from build123d import *

# Parameters (mm, degrees)
SKETCH001_R     = 6
POCKET_DEPTH    = 5.020854
CHAMFER_SIZE    = 0.25
CHAMFER001_SIZE = 1


with BuildPart() as pocket:
    # Sketch003 → Revolution001 (revolve)
    with BuildSketch(Plane.XZ):
        Polygon((0, -4.019854), (5, -2.2), (5, 1), (0, 1), align=None)
    revolve(axis=Axis((0, 0, 0), (0, 0, 1)))

    # Sketch001 → Pocket (cut, through all)
    with BuildSketch(Plane(origin=(0, 0, 1), x_dir=(-1, 0, 0), z_dir=(0, 0, 1))):
        Circle(SKETCH001_R)
        Polygon((-1.443376, 2.5), (1.443376, 2.5), (2.886751, 0), (1.443376, -2.5), (-1.443376, -2.5), (-2.886751, 0), align=None, mode=Mode.SUBTRACT)
    extrude(amount=-POCKET_DEPTH, mode=Mode.SUBTRACT)


with BuildPart() as chamfer001:
    # Sketch → Revolution (revolve)
    with BuildSketch(Plane.XZ):
        Polygon((2.88675, 0), (6.719999, 0), (3, -3.72), (3, -12), (0, -12), (0, -2.886753), align=None)
    revolve(axis=Axis((0, 0, 0), (0, 0, 1)))

    # Cut: cut Pocket
    add(pocket.part, mode=Mode.SUBTRACT)

    # Chamfer
    chamfer_edges = [chamfer001.edges().sort_by_distance(p)[0] for p in [
        (-6.719999, 0, 0),
    ]]
    chamfer(chamfer_edges, length=CHAMFER_SIZE)

    # Chamfer001
    chamfer001_edges = [chamfer001.edges().sort_by_distance(p)[0] for p in [
        (-3, 0, -12),
    ]]
    chamfer(chamfer001_edges, length=CHAMFER001_SIZE)


solid = chamfer001.part
Could you check a few things on this model? Use its own coordinates, in mm. A direction names the side the tool comes from. Give positions to 0.01 mm unless a question says otherwise; leave off trailing zeros. Order: outer loops, then holes, each group sorted by start corner. A loop starts at its lowest first (then second) coordinate and runs counter-clockwise, first axis right, second up. Notation, with made-up numbers: (71, 51.25) - (118, 51.25) arc R25 ccw to (118, 72.25) - close; hole circle Ø2 at (61.5, 43). An arc over 180 degrees is marked (long way). One line per question, with ' | ' between items. Start each with the question number.
Item 1: I'm going to push flat-ended pins straight in: pin 1 Ø4 at (y, z) = (-0.5, -10) entering from -X; pin 2 Ø1 at (y, z) = (2, -1.5) entering from -X; pin 3 Ø1.5 at (x, z) = (2, -3.5) entering from -Y. Where does each tip first touch, or does it pass through?
Item 2: I want a section at B-B on z = -9.75. Write out the boundary of the cut face in (x, y).
Item 3: I want a section at A-A on z = -2.25. Write out the boundary of the cut face in (x, y).
Item 4: For faces 1 (the flat face through (-2.175, 1.233, -1.533)), 2 (the cylindrical face through (-3, 0, -7)), 3 (the flat face through (-3, -1, 0)), which set-ups out of +Z, -Z, +X, -X, +Y, -Y let a thin tool reach every point of the face, with its end or its side?
Item 5: I need wall thicknesses on probe 1 along X at (y, z) = (-0.25, -1.75); probe 2 along Y at (x, z) = (0, -10.5); probe 3 along Z at (x, y) = (-3.75, 0). Which ranges of each line are inside material? Lowest first, please. Write a range as [from, to].
Item 6: Thinking about a two-plate mould opening in X: for faces 4 (the flat face through (0, 0, -12)), 5 (the conical face through (0.172, 0.054, -3.954)), 6 (the conical face through (1.464, -2.814, -3.548)), which applies, pulls with the +X half, pulls with the -X half, needs draft (parallel to the pull), parting line crosses it, or undercut?
Verdict:
1) pin 1: x = -3 | pin 2: x = -5.39 | pin 3: y = -3.52
2) outline: circle Ø6 at (0, 0)
3) outline: circle Ø8.94 at (0, 0); hole (-2.89, 0) - (-1.44, -2.5) - (1.44, -2.5) - (2.89, 0) - (1.44, 2.5) - (-1.44, 2.5) - close
4) face 1: +Z | face 2: -Z | face 3: +Z, +X, -X, +Y, -Y
5) probe 1: [-4.96, -2.74], [2.74, 4.96] | probe 2: [-3, 3] | probe 3: [-2.97, 0]
6) face 4: needs draft | face 5: undercut | face 6: parting line crosses it
